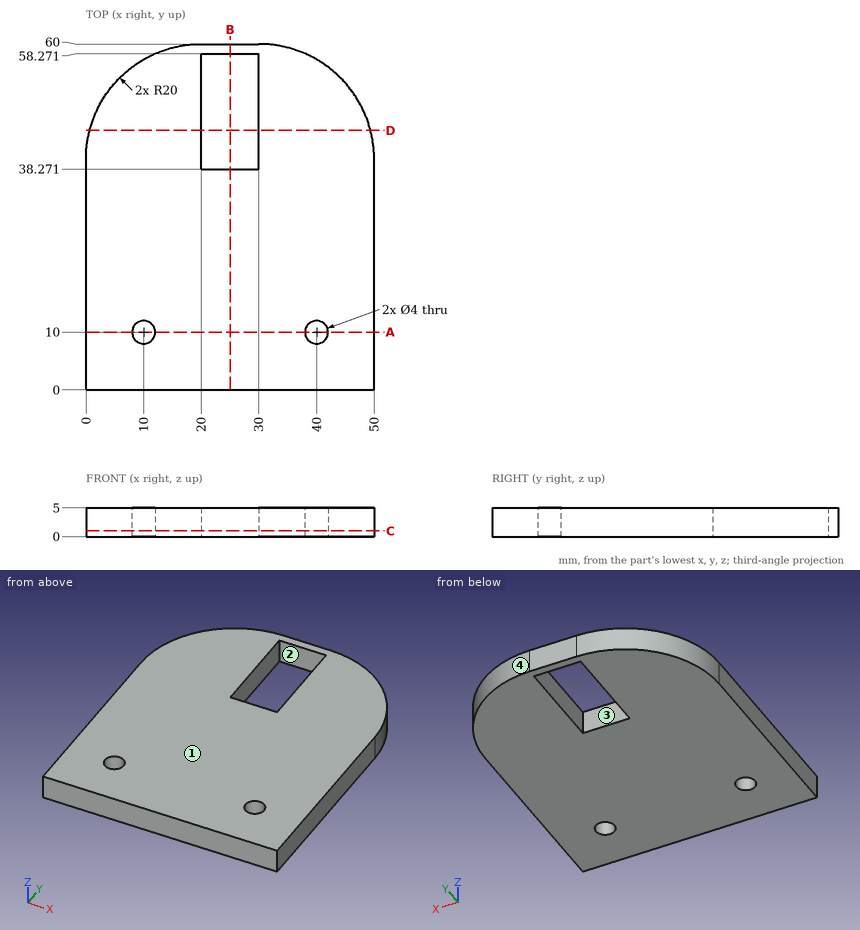
Geometry check sheet. Reference: drawing and pictorial views, mm from the part's lowest x, y, z. Give positions to 0.01 mm unless a question says otherwise; leave off trailing zeros. Write each loop counter-clockwise with the first axis right and the second up, starting at its lowest first coordinate (ties: lowest second). Pieces come first, ordered by that corner, then holes. Notation, with made-up numbers: M 82,82.5 L 96,82.5 A18 cw 96,115.5 Z; hole C 31.5,-31 d3. An arc over 180 degrees is marked long. Put each result on its own line as item: value. Start each with the question number.
1. Section check D-D (y = 45). Record the cut outline in (x, z) (1 decimal).
2. Section check C-C (z = 1). Record the cut outline in (x, y), and give its area (3 significant figures).
3. Scan lines: line 1 along X through (y, z) = (40, 1.2); line 2 along X through (y, z) = (45.5, 4.65); line 3 along Y through (x, z) = (10, 1.35). Record each from-to range of solid material in increasing order. Write a range as [from, to].
4. Draft check along X on the marked faces 1, 2, 3 and 4. Enter one of: +X half, -X half, draft (parallel to the pull), parting line (faces both ways), or undercut.
5. Section check B-B (x = 25). Record the cut outline in (y, z), and give its area (3 significant figures).
6. Section check A-A (y = 10). Record the cut outline in (x, z), and give its area (3 significant figures).
7. Go/stop test with flat-tipped pins: pin 1 Ø4.5 at (x, y) = (40, 10) entering from -Z; pin 2 Ø2.5 at (y, z) = (53, 2) entering from +X (1 decimal); pin 3 Ø1.5 at (x, z) = (44.5, 2) entering from +Y (1 decimal); pin 4 Ø3 at (x, z) = (15, 4) entering from +Y. Record where each tip stops, or that it passes through.
Answer list:
1. outline: M 0.6,0 L 20,0 L 20,5 L 0.6,5 Z; M 30,0 L 49.4,0 L 49.4,5 L 30,5 Z
2. outline: M 0,0 L 50,0 L 50,40 A20 ccw 30,60 L 20,60 A20 ccw 0,40 Z; hole C 10,10 d4; hole M 20,38.27 L 30,38.27 L 30,58.27 L 20,58.27 Z; hole C 40,10 d4
2. area: 2,600 mm2
3. line 1: [0, 20], [30, 50]
3. line 2: [0.77, 20], [30, 49.23]
3. line 3: [0, 8], [12, 57.32]
4. face 1: draft
4. face 2: undercut
4. face 3: undercut
4. face 4: +X half
5. outline: M 0,0 L 38.27,0 L 38.27,5 L 0,5 Z; M 58.27,0 L 60,0 L 60,5 L 58.27,5 Z
5. area: 200 mm2
6. outline: M 0,0 L 8,0 L 8,5 L 0,5 Z; M 12,0 L 38,0 L 38,5 L 12,5 Z; M 42,0 L 50,0 L 50,5 L 42,5 Z
6. area: 210 mm2
7. pin 1: z = 0
7. pin 2: x = 46.2
7. pin 3: y = 54.5
7. pin 4: y = 59.69
